```python
from build123d import *

# Parameters (mm, degrees)
BOSS_EXTRUDE1_DEPTH = 24
SKETCH2_W           = 8.2
SKETCH2_H           = 5
CUT_EXTRUDE1_DEPTH  = 3
SKETCH4_W           = 0.5
SKETCH4_H           = 5
CUT_EXTRUDE2_DEPTH  = 0.5
SKETCH5_R           = 1.3
BOSS_EXTRUDE2_DEPTH = 10


with BuildPart() as part:
    # Sketch1 → Boss-Extrude1 (new body)
    with BuildSketch(Plane(origin=(0, 0, 0), x_dir=(0, 0, -1), z_dir=(1, 0, 0))):
        with BuildLine():
            Line((-1.4, 2.7), (1.4, 2.7))
            Line((1.4, 2.7), (1.4, 1.428285686))
            ThreePointArc((1.4, 1.428285686), (0, -2), (-1.4, 1.428285686))
            Line((-1.4, 1.428285686), (-1.4, 2.7))
        make_face()
    extrude(amount=BOSS_EXTRUDE1_DEPTH)

    # Sketch2 → Cut-Extrude1 (cut)
    with BuildSketch(Plane(origin=(0, 2.7, 0), x_dir=(1, 0, 0), z_dir=(0, 1, 0))):
        Rectangle(SKETCH2_W, SKETCH2_H)
    extrude(amount=-CUT_EXTRUDE1_DEPTH, mode=Mode.SUBTRACT)

    # Sketch3 → Revolve1 (revolve)
    with BuildSketch(Plane.XY):
        Polygon((0.074999, 0.499998), (1.224998, 0.499998), (1.224998, 0.7), (-0.075005, 0.7), (-0.075005, 1.58), (0.445, 2.099999), (0.445, 2.599999), (2, 2.599999), (2, -0.3), (0.074999, -0.3), align=None)
    revolve(axis=Axis((2, 2.599999, 0), (0, -1, 0)))

    # Sketch4 → Cut-Extrude2 (cut)
    with BuildSketch(Plane(origin=(0, 2.599999, 0), x_dir=(1, 0, 0), z_dir=(0, 1, 0))):
        with Locations((2, 0)):
            Rectangle(SKETCH4_W, SKETCH4_H)
    extrude(amount=-CUT_EXTRUDE2_DEPTH, mode=Mode.SUBTRACT)

    # Sketch5 → Boss-Extrude2 (add)
    with BuildSketch(Plane(origin=(24, 0, 0), x_dir=(0, 0, -1), z_dir=(1, 0, 0))):
        Circle(SKETCH5_R)
    extrude(amount=BOSS_EXTRUDE2_DEPTH)


solid = part.part
```
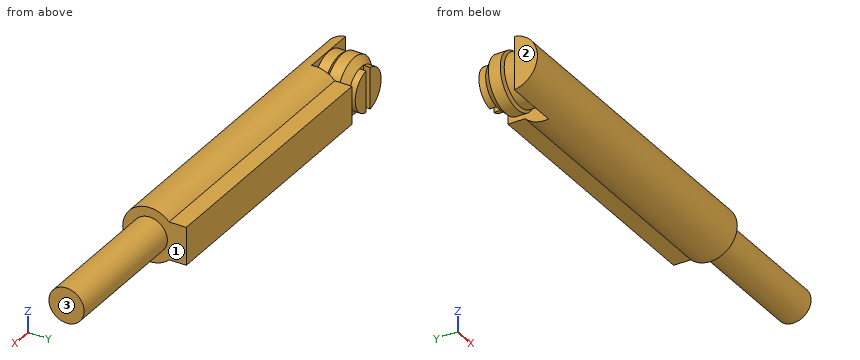
Part model, mm, in its own coordinate system. Face numbers are marked on the shaded views. A direction names the side the tool comes from. Round coordinates to 2 decimals unless told otherwise and drop trailing zeros. Loops run counter-clockwise (first coordinate to the right, second up) from the corner with the lowest first, then second, coordinate; pieces in that order, holes last. Notation, with made-up numbers: (33.5, 59.5) -> (48.5, 59.5) arc R18 ccw to (48.5, 85.5) -> close; hole circle Ø5 at (32, -32). An arc over 180 degrees is marked (long way). Use a Markdown table: item, result.
1) Cut at D-D, the plane x = 6. List the corners of the cut face in (y, z), and give its area (3 significant figures).
The answers:
| item | result |
|---|---|
| outline | (1.43, -1.4) -> (2.7, -1.4) -> (2.7, 1.4) -> (1.43, 1.4) arc R2 ccw (long way) to start |
| area | 15.0 mm2 |
2) Drop flat-ended pins along their axis: pin 1 Ø1.9 at (x, z) = (2, 0) entering from +Y; pin 2 Ø0.6 at (y, z) = (2.5, -0.5) entering from -X; pin 3 Ø2 at (x, z) = (6, 1.5) entering from +Y; pin 4 Ø1 at (x, y) = (11, 2) entering from -Z. Give the stop position or say it passes through.
The answers:
| item | result |
|---|---|
| pin 1 | stops at y = 2.6 |
| pin 2 | stops at x = 0.46 |
| pin 3 | stops at y = 2.7 |
| pin 4 | stops at z = -1.4 |
3) Tool access for the marked faces 1, 2 and 3: list every direction of +Z, -Z, +X, -X, +Y, -Y with a clear straight run to the whole face (end or side of a thin tool).
The answers:
| item | result |
|---|---|
| face 1 | +X |
| face 2 | +Z, -Z, -X, -Y |
| face 3 | +Z, -Z, +X, +Y, -Y |
4) Cut at A-A, the plane y = 0. List the corners of the cut face in (x, z) (3 decimals).
The answers:
| item | result |
|---|---|
| outline | circle Ø3.85 at (2, 0); (4.1, -2) -> (24, -2) -> (24, -1.3) -> (34, -1.3) -> (34, 1.3) -> (24, 1.3) -> (24, 2) -> (4.1, 2) -> close |
5) Probe line 1 (X direction, y = -0.75, z = -1); line 2 (Z direction, x = 14, y = 1.9); line 3 (X direction, y = 0.6, z = -0.4). List the from-to ranges inside material, lowest first. Write a range as [from, to].
The answers:
| item | result |
|---|---|
| line 1 | x = [0, 34] |
| line 2 | z = [-1.4, 1.4] |
| line 3 | x = [1.34, 2.66], [4.1, 34] |
6) Cut at C-C, the plane x = 31. List the corners of the cut face in (y, z).
The answers:
| item | result |
|---|---|
| outline | circle Ø2.6 at (0, 0) |
